from build123d import *

# Parameters (mm, degrees)
F0_R     = 4.7625
F0_R_2   = 2.159
F1_DEPTH = 9.525
F2_DEPTH = 5.08
F3_R     = 3.302
F4_DEPTH = 6.35


with BuildPart() as f1:
    # F0 (on Top) → F1 (new body)
    with BuildSketch(Plane.XY):
        Circle(F0_R)
        Circle(F0_R_2, mode=Mode.SUBTRACT)
        Circle(F0_R_2)
    extrude(amount=F1_DEPTH)

    # F0 (on Top) → F2 (join)
    with BuildSketch(Plane.XY):
        Circle(F0_R_2)
    extrude(amount=-F2_DEPTH)

    # F3 (on face) → F4 (cut)
    with BuildSketch(Plane.XY.offset(9.525)):
        Circle(F3_R)
    extrude(amount=-F4_DEPTH, mode=Mode.SUBTRACT)


solid = f1.part
Verification items for the finished model (mm, model axes). A direction names the side the tool comes from. Coordinates: 2 decimals unless noted, no trailing zeros. Order: outer loops, then holes, each group sorted by start corner. A loop starts at its lowest first (then second) coordinate and runs counter-clockwise, first axis right, second up. Notation, with made-up numbers: M 30,-39 L 43,-39 A33 cw 43,-11 Z; hole C 45,14 d3. An arc over 180 degrees is marked long. One line per item, written item: value. Start each with the question number.
Item 1: Gauge pin test, flat ends, axial feed: pin 1 (3 mm diameter, centred on x = 0, y = 1.5, fed in from +Z) (3 decimals); pin 2 (1 mm diameter, centred on y = -1, z = 0, fed in from -X); pin 3 (2 mm diameter, centred on x = -1.5, z = 2.5, fed in from +Y). Record the tip position at first contact, or that the pin passes through.
Item 2: Sectioned sample at A-A (y = 0). Enter the section's corners in (x, z) (1 decimal).
Item 3: Sectioned sample at C-C (x = -0.5). Enter the section's corners in (y, z) (3 decimals), then the cut area to 3 significant figures.
Item 4: Scan lines: probe 1 along Y at (x, z) = (0, 7.5); probe 2 along Z at (x, y) = (2, 1) (3 decimals); probe 3 along X at (y, z) = (2.75, 4.5). Record each from-to range of solid material in increasing order.
Item 5: Access from +Z, -Z, +X, -X, +Y, -Y to the whole of each face (thin tool, end or side, straight path). Record for faces 1 (the cylindrical face through (-0.28, 2.14, -2.5)), 2 (the cylindrical face through (3.05, -1.26, 6.39)), 3 (the flat face through (0, 0, -5.08)).
Item 6: Mould release check, pull along X, two halves, no side actions. Record for faces 4 (the flat face through (0, 0, 3.175)), 5 (the cylindrical face through (-3.78, -2.9, 4.7)), 6 (the flat face through (2.05, 1.13, 0)): released by +X, released by -X, zero draft, split by the parting line, or undercut.
Item 7: Sectioned sample at B-B (z = 7.5). Enter the section's corners in (x, y) (1 decimal).
Item 8: Sectioned sample at D-D (z = 2.75). Enter the section's corners in (x, y) (1 decimal), then the cut area to 3 significant figures.
Conclusion:
1. pin 1: stops at z = 3.175
1. pin 2: stops at x = -4.74
1. pin 3: stops at y = 4.74
2. outline: M -4.8,0 L -2.2,0 L -2.2,-5.1 L 2.2,-5.1 L 2.2,0 L 4.8,0 L 4.8,9.5 L 3.3,9.5 L 3.3,3.2 L -3.3,3.2 L -3.3,9.5 L -4.8,9.5 Z
3. outline: M -4.736,0 L -2.1,0 L -2.1,-5.08 L 2.1,-5.08 L 2.1,0 L 4.736,0 L 4.736,9.525 L 3.264,9.525 L 3.264,3.175 L -3.264,3.175 L -3.264,9.525 L -4.736,9.525 Z
3. area: 70.1 mm^2
4. probe 1: y = -4.76 to -3.3, 3.3 to 4.76
4. probe 2: z = 0 to 3.175
4. probe 3: x = -3.89 to -1.83, 1.83 to 3.89
5. face 1: -Z
5. face 2: +Z
5. face 3: -Z, +X, -X, +Y, -Y
6. face 4: undercut
6. face 5: split by the parting line
6. face 6: zero draft
7. outline: C 0,0 d9.5; hole C 0,0 d6.6
8. outline: C 0,0 d9.5
8. area: 71.3 mm^2
